Verification items for this drawing (mm, ordinates from the low corner). A direction names the side the tool comes from. Round coordinates to 2 decimals unless told otherwise and drop trailing zeros. Order: outer loops, then holes, each group sorted by start corner. A loop starts at its lowest first (then second) coordinate and runs counter-clockwise, first axis right, second up. Notation, with made-up numbers: (-7, -6.5) -> (17, -6.5) arc R23 ccw to (17, 12.5) -> close; hole circle Ø10 at (-25, 55). An arc over 180 degrees is marked (long way). Return JSON: item names as keys, results as strings. Group by question number.
Item 1: Depth check by flat-ended pin: pin 1 Ø5 at (y, z) = (4.5, 10) entering from +X; pin 2 Ø5 at (x, y) = (80.5, 3) entering from +Z; pin 3 Ø1.5 at (x, z) = (33.5, 19) entering from +Y. Enter the tip coordinate at first touch or a pass-through.
Item 2: Sectioned sample at C-C on y = 31.5. Record the cut outline in (x, z).
Item 3: Sectioned sample at A-A on x = 109. Record the cut outline in (y, z), plus the area to 3 significant figures.
Item 4: Sectioned sample at B-B on z = 8. Record the cut outline in (x, y).
Item 5: Access from +Z, -Z, +X, -X, +Y, -Y to the whole of each face (thin tool, end or side, straight path). Record for the marked faces 1, 2 and 3.
Item 6: Scan lines: probe 1 along Z at (x, y) = (47.5, 6.5); probe 2 along Y at (x, z) = (26, 14.5); probe 3 along X at (y, z) = (29.5, 2.75). Record each from-to range of solid material in increasing order. Write a range as from..to.
Item 7: Sectioned sample at D-D on x = 132. Record the cut outline in (y, z), plus the area to 3 significant figures.
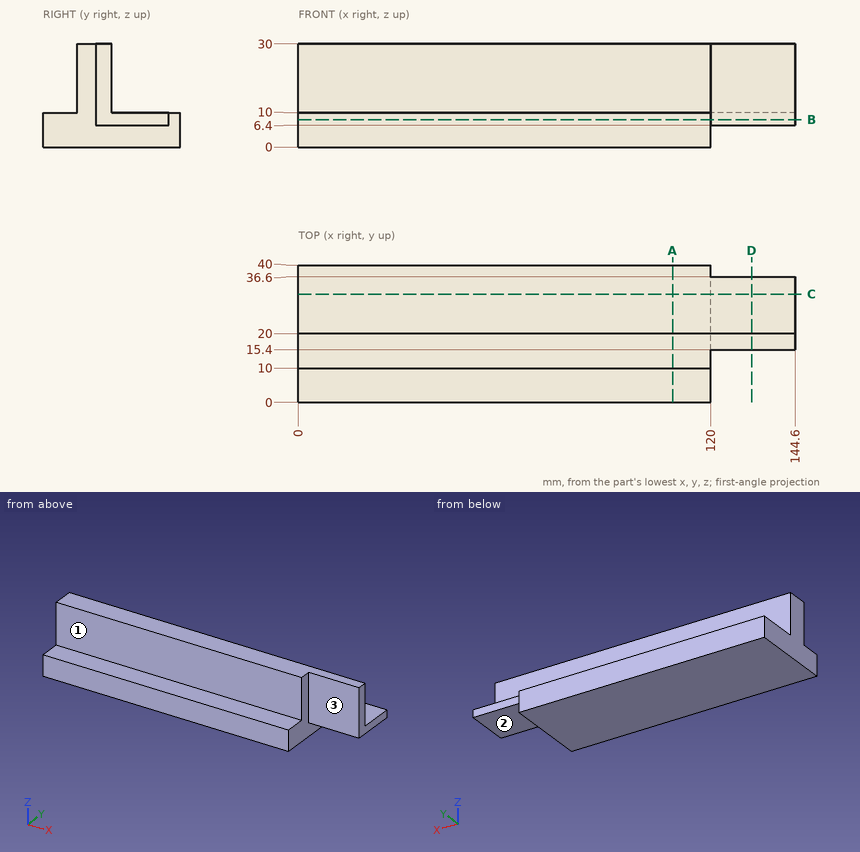
Recorded:
{
 "1": {"pin 1": "x = 120", "pin 2": "z = 10", "pin 3": "y = 20"},
 "2": {"outline": "(0, 0) -> (120, 0) -> (120, 6.4) -> (144.6, 6.4) -> (144.6, 10) -> (0, 10) -> close"},
 "3": {"outline": "(0, 0) -> (40, 0) -> (40, 10) -> (20, 10) -> (20, 30) -> (10, 30) -> (10, 10) -> (0, 10) -> close", "area": "600 mm²"},
 "4": {"outline": "(0, 0) -> (120, 0) -> (120, 15.4) -> (144.6, 15.4) -> (144.6, 36.6) -> (120, 36.6) -> (120, 40) -> (0, 40) -> close"},
 "5": {"face 1": "+Z, +X, -X, -Y", "face 2": "-Z, +X, +Y, -Y", "face 3": "+Z, -Z, +X, -Y"},
 "6": {"probe 1": "0..10", "probe 2": "10..20", "probe 3": "0..120"},
 "7": {"outline": "(15.4, 6.4) -> (36.6, 6.4) -> (36.6, 10) -> (20, 10) -> (20, 30) -> (15.4, 30) -> close", "area": "168 mm²"}
}
